Can you work these out from the model? Positions are in its coordinate system, mm. A direction names the side the tool comes from. Give positions to 0.01 mm unless a question says otherwise; leave off trailing zeros. Loops run counter-clockwise (first coordinate to the right, second up) from the corner with the lowest first, then second, coordinate; pieces in that order, holes last. Notation, with made-up numbers: M -10.5,87.5 L 8.5,87.5 A21 cw 8.5,111.5 Z; hole C -3.75,55.25 d1. An arc over 180 degrees is marked long. Put each result on its own line as item: value. Start each with the question number.
1) For faces 4 (the flat face through (-17, 331, 469.163)), 5 (the flat face through (-16, -498.963, -6)), 6 (the flat face through (-31.937, 327, 453)), which set-ups out of +Z, -Z, +X, -X, +Y, -Y let a thin tool reach every point of the face, with its end or its side?
2) Imagine slicing it at B-B (z = -13.5). Write out the boundary of the cut face in (x, y), then the cut area to 3 significant figures.
3) Imagine slicing it at C-C (y = -276.5). Write out the boundary of the cut face in (x, z).
4) If we mould it in two halves opening along Y, with no side actions, what happens to faces 1 (the flat face through (-1.737, -104, -6)), 2 (the flat face through (-16, -500.7, -6)), 3 (the flat face through (-17, 331, 470.9))? For each: +Y half, -Y half, draft (parallel to the pull), parting line (faces both ways), or undercut.
5) Imagine slicing it at A-A (x = -16.5). Write out the boundary of the cut face in (y, z), then the cut area to 3 significant figures.
6) Please list where these lines run through material, in increasing order: line 1 along Y through (x, z) = (-10, 94); line 2 along Y through (x, z) = (-27.5, 109); line 3 along X through (y, z) = (-180.5, -200.5). Write a range as from..to.
7) For P1, Ø8.5, axis at x = -22, y = 356, coming from the -Z side; P2, Ø1.7, axis at x = -19.5, y = -499, coming from the -Z side; P3, Ø1, axis at x = -0.5, z = -469, coming from the -Y side, each with a flat end and sliding along its axis, tell me the tip position at first contact or that it passes through.
from build123d import *

# Parameters (mm, degrees)
BASE_FLANGE2_DEPTH            = 1.7366
EDGE_FLANGE5_STRIP_W          = 8.4196
EDGE_FLANGE5_STRIP_H          = 1.7366
EDGE_FLANGE5_STRIP_CUT_DEPTH  = 939.6
EDGE_FLANGE5_RELIEF_W         = 9.2879
EDGE_FLANGE5_RELIEF_H         = 0.8683
EDGE_FLANGE5_RELIEF_CUT_DEPTH = 1.7366
EDGE_FLANGE5_DEPTH            = 939.6
EDGE_FLANGE6_STRIP_W          = 8.4196
EDGE_FLANGE6_STRIP_H          = 1.7366
EDGE_FLANGE6_STRIP_CUT_DEPTH  = 284.5
EDGE_FLANGE6_RELIEF_W         = 9.2879
EDGE_FLANGE6_RELIEF_H         = 0.8683
EDGE_FLANGE6_RELIEF_CUT_DEPTH = 1.7366
EDGE_FLANGE6_DEPTH            = 284.5
EDGE_FLANGE8_STRIP_W          = 8.4196
EDGE_FLANGE8_STRIP_H          = 1.7366
EDGE_FLANGE8_STRIP_CUT_DEPTH  = 874.9634
EDGE_FLANGE8_RELIEF_W         = 9.2879
EDGE_FLANGE8_RELIEF_H         = 0.8683
EDGE_FLANGE8_RELIEF_CUT_DEPTH = 1.7366
EDGE_FLANGE8_DEPTH            = 874.9634
EDGE_FLANGE9_STRIP_W          = 8.4196
EDGE_FLANGE9_STRIP_H          = 1.7366
EDGE_FLANGE9_STRIP_CUT_DEPTH  = 284.3634
EDGE_FLANGE9_RELIEF_W         = 9.2879
EDGE_FLANGE9_RELIEF_H         = 0.8683
EDGE_FLANGE9_RELIEF_CUT_DEPTH = 1.7366
EDGE_FLANGE9_DEPTH            = 284.3634


# Sheet-metal steps are written as plain solids
with BuildPart() as part:
    # Sketch10 → Base-Flange2 (new body)
    with BuildSketch(Plane(origin=(0, 0, 0), x_dir=(0, 0, -1), z_dir=(1, 0, 0))):
        Polygon((-470.9, 501), (-470.9, 184.3), (499, 184.3), (499, -500.7), (-501, -500.7), (-501, 501), align=None)
    extrude(amount=-BASE_FLANGE2_DEPTH)

    # Edge-Flange5 strip (across the edge) → Edge-Flange5 strip cut (cut)
    with BuildSketch(Plane(origin=(-1.7366, -500.7, -468.8), x_dir=(0, 1, 0), z_dir=(0, 0, 1))):
        with Locations((-1.7366, -0.8683)):
            Rectangle(EDGE_FLANGE5_STRIP_W, EDGE_FLANGE5_STRIP_H)
    extrude(amount=EDGE_FLANGE5_STRIP_CUT_DEPTH, mode=Mode.SUBTRACT)

    # Edge-Flange5 relief (on the sheet) → Edge-Flange5 relief cut (cut)
    with BuildSketch(Plane(origin=(-1.7366, -498.2268, -468.8), x_dir=(0, 1, 0), z_dir=(-1, 0, 0))):
        with Locations((-3.77565, 0.43415)):
            Rectangle(EDGE_FLANGE5_RELIEF_W, EDGE_FLANGE5_RELIEF_H)
        with Locations((-3.77565, -940.03415)):
            Rectangle(EDGE_FLANGE5_RELIEF_W, EDGE_FLANGE5_RELIEF_H)
    extrude(amount=-EDGE_FLANGE5_RELIEF_CUT_DEPTH, mode=Mode.SUBTRACT)

    # Edge-Flange5 section (across the edge) → Edge-Flange5 (add)
    with BuildSketch(Plane(origin=(-1.7366, -500.7, -468.8), x_dir=(0, 1, 0), z_dir=(0, 0, 1))):
        with BuildLine():
            Line((0, 0.7366), (0, 28.2634))
            Line((0, 28.2634), (1.7366, 28.2634))
            Line((1.7366, 28.2634), (1.7366, 0.7366))
            ThreePointArc((1.7366, 0.7366), (1.952345145, 0.215745145), (2.4732, 0))
            Line((2.4732, 0), (2.4732, -1.7366))
            ThreePointArc((2.4732, -1.7366), (0.724383509, -1.012216491), (0, 0.7366))
        make_face()
    extrude(amount=EDGE_FLANGE5_DEPTH)

    # Edge-Flange6 strip (across the edge) → Edge-Flange6 strip cut (cut)
    with BuildSketch(Plane(origin=(-1.7366, 470.8, 470.9), x_dir=(0, 0, 1), z_dir=(0, -1, 0))):
        with Locations((-3.4732, -0.8683)):
            Rectangle(EDGE_FLANGE6_STRIP_W, EDGE_FLANGE6_STRIP_H)
    extrude(amount=EDGE_FLANGE6_STRIP_CUT_DEPTH, mode=Mode.SUBTRACT)

    # Edge-Flange6 relief (on the sheet) → Edge-Flange6 relief cut (cut)
    with BuildSketch(Plane(origin=(-1.7366, 470.8, 471.6366), x_dir=(0, 0, 1), z_dir=(-1, 0, 0))):
        with Locations((-3.77565, 0.43415)):
            Rectangle(EDGE_FLANGE6_RELIEF_W, EDGE_FLANGE6_RELIEF_H)
        with Locations((-3.77565, -284.93415)):
            Rectangle(EDGE_FLANGE6_RELIEF_W, EDGE_FLANGE6_RELIEF_H)
    extrude(amount=-EDGE_FLANGE6_RELIEF_CUT_DEPTH, mode=Mode.SUBTRACT)

    # Edge-Flange6 section (across the edge) → Edge-Flange6 (add)
    with BuildSketch(Plane(origin=(-1.7366, 470.8, 470.9), x_dir=(0, 0, 1), z_dir=(0, -1, 0))):
        with BuildLine():
            Line((-1.7366, 0.7366), (-1.7366, 30.2))
            Line((-1.7366, 30.2), (0, 30.2))
            Line((0, 30.2), (0, 0.7366))
            ThreePointArc((0, 0.7366), (0.215745145, 0.215745145), (0.7366, 0))
            Line((0.7366, 0), (0.7366, -1.7366))
            ThreePointArc((0.7366, -1.7366), (-1.012216491, -1.012216491), (-1.7366, 0.7366))
        make_face()
    extrude(amount=EDGE_FLANGE6_DEPTH)

    # Edge-Flange8 strip (across the edge) → Edge-Flange8 strip cut (cut)
    with BuildSketch(Plane(origin=(-1.7366, 184.3, 408.1634), x_dir=(0, -1, 0), z_dir=(0, 0, -1))):
        with Locations((-3.4732, -0.8683)):
            Rectangle(EDGE_FLANGE8_STRIP_W, EDGE_FLANGE8_STRIP_H)
    extrude(amount=EDGE_FLANGE8_STRIP_CUT_DEPTH, mode=Mode.SUBTRACT)

    # Edge-Flange8 relief (on the sheet) → Edge-Flange8 relief cut (cut)
    with BuildSketch(Plane(origin=(-1.7366, 183.5634, 408.1634), x_dir=(0, -1, 0), z_dir=(-1, 0, 0))):
        with Locations((-3.77565, 0.43415)):
            Rectangle(EDGE_FLANGE8_RELIEF_W, EDGE_FLANGE8_RELIEF_H)
        with Locations((-3.77565, -875.39755)):
            Rectangle(EDGE_FLANGE8_RELIEF_W, EDGE_FLANGE8_RELIEF_H)
    extrude(amount=-EDGE_FLANGE8_RELIEF_CUT_DEPTH, mode=Mode.SUBTRACT)

    # Edge-Flange8 section (across the edge) → Edge-Flange8 (add)
    with BuildSketch(Plane(origin=(-1.7366, 184.3, 408.1634), x_dir=(0, -1, 0), z_dir=(0, 0, -1))):
        with BuildLine():
            Line((-1.7366, 0.7366), (-1.7366, 20))
            Line((-1.7366, 20), (0, 20))
            Line((0, 20), (0, 0.7366))
            ThreePointArc((0, 0.7366), (0.215745145, 0.215745145), (0.7366, 0))
            Line((0.7366, 0), (0.7366, -1.7366))
            ThreePointArc((0.7366, -1.7366), (-1.012216491, -1.012216491), (-1.7366, 0.7366))
        make_face()
    extrude(amount=EDGE_FLANGE8_DEPTH)

    # Edge-Flange9 strip (across the edge) → Edge-Flange9 strip cut (cut)
    with BuildSketch(Plane(origin=(-31.9366, 186.4366, 469.1634), x_dir=(1, 0, 0), z_dir=(0, 1, 0))):
        with Locations((-3.4732, -0.8683)):
            Rectangle(EDGE_FLANGE9_STRIP_W, EDGE_FLANGE9_STRIP_H)
    extrude(amount=EDGE_FLANGE9_STRIP_CUT_DEPTH, mode=Mode.SUBTRACT)

    # Edge-Flange9 relief (on the sheet) → Edge-Flange9 relief cut (cut)
    with BuildSketch(Plane(origin=(-31.2, 186.4366, 469.1634), x_dir=(1, 0, 0), z_dir=(0, 0, -1))):
        with Locations((-3.77565, 0.43415)):
            Rectangle(EDGE_FLANGE9_RELIEF_W, EDGE_FLANGE9_RELIEF_H)
    extrude(amount=-EDGE_FLANGE9_RELIEF_CUT_DEPTH, mode=Mode.SUBTRACT)

    # Edge-Flange9 section (across the edge) → Edge-Flange9 (add)
    with BuildSketch(Plane(origin=(-31.9366, 186.4366, 469.1634), x_dir=(1, 0, 0), z_dir=(0, 1, 0))):
        with BuildLine():
            Line((-1.7366, 0.7366), (-1.7366, 30.2))
            Line((-1.7366, 30.2), (0, 30.2))
            Line((0, 30.2), (0, 0.7366))
            ThreePointArc((0, 0.7366), (0.215745145, 0.215745145), (0.7366, 0))
            Line((0.7366, 0), (0.7366, -1.7366))
            ThreePointArc((0.7366, -1.7366), (-1.012216491, -1.012216491), (-1.7366, 0.7366))
        make_face()
    extrude(amount=EDGE_FLANGE9_DEPTH)


solid = part.part
Recorded:
1. face 4: -Z, +X, +Y
1. face 5: +Z, -Z, -X
1. face 6: -Z, +X, +Y, -Y
2. outline: M -30,-500.7 L -2.47,-500.7 A2.47 ccw 0,-498.23 L 0,183.56 A2.47 ccw -2.47,186.04 L -21.74,186.04 L -21.74,184.3 L -2.47,184.3 A0.74 cw -1.74,183.56 L -1.74,-498.23 A0.74 cw -2.47,-498.96 L -30,-498.96 Z
2. area: 1,270 mm²
3. outline: M -1.74,-499 L 0,-499 L 0,501 L -1.74,501 Z
4. face 1: undercut
4. face 2: -Y half
4. face 3: draft
5. outline: M -500.7,-468.8 L -498.96,-468.8 L -498.96,470.8 L -500.7,470.8 Z; M 184.3,-466.8 L 186.04,-466.8 L 186.04,408.16 L 184.3,408.16 Z; M 186.3,469.16 L 470.8,469.16 L 470.8,470.9 L 186.3,470.9 Z
5. area: 3,650 mm²
6. line 1: -500.7..-498.96, 184.3..186.04
6. line 2: -500.7..-498.96
6. line 3: -1.74..0
7. P1: z = 469.16
7. P2: z = -468.8
7. P3: y = -500.18
